Part model, mm, in its own coordinate system. A direction names the side the tool comes from. Give positions to 0.01 mm unless a question says otherwise; leave off trailing zeros. Write each loop counter-clockwise with the first axis right and the second up, starting at its lowest first coordinate (ties: lowest second). Pieces come first, ordered by that corner, then holes. Notation, with made-up numbers: (57, -34.5) - (74, -34.5) arc R16 cw to (74, -15.5) - close; hole circle Ø11 at (59.5, 86.5). An arc over 180 degrees is marked (long way). Answer in a Markdown table with one row per item. Add a question column.
1. Band-saw the part on D-D on z = 5. Write the cut outline in (x, y), plus the area to 3 significant figures.
2. Which spindle directions (+Z, -Z, +X, -X, +Y, -Y) get a long thin tool onto all of the face, cutting with end or side? Do faces 1 (the cylindrical face through (91.515, -6.601, 1.578)), 2 (the flat face through (83, -6, 5.8)). Say none if no direction does.
3. Drop flat-ended pins along their axis: pin 1 Ø1 at (x, y) = (89.5, -6.5) entering from -Z; pin 2 Ø3 at (y, z) = (-7.5, 3) entering from +X; pin 3 Ø3 at (y, z) = (-2.5, 2.5) entering from -X; pin 4 Ø6.5 at (x, y) = (85.21, -1.76) entering from +Z. Give the stop position or say it passes through.
4. Probe line 1 along X through (y, z) = (-1.75, 3.6); line 2 along Y through (x, z) = (84.25, 0.3); line 3 along X through (y, z) = (5.5, 1). List the from-to ranges inside material, lowest first.
5. Band-saw the part on C-C on z = 1.45. Write the cut outline in (x, y).
6. Pull direction Y, two halves, no side cores. Call faces 3 (the cylindrical face through (81.21, -1.59, 4.26)), 4 (the cylindrical face through (93.75, -5.31, 2.86)), 5 (the flat face through (88, 6, 0)): released by +Y, released by -Y, zero draft, split by the parting line, or undercut.
7. Band-saw the part on A-A on x = 79. Write the cut outline in (y, z).
8. Band-saw the part on B-B on y = 5.25. Write the cut outline in (x, z).
```python
from build123d import *

# Parameters (mm, degrees)
SKETCH1_R           = 9.25
BOSS_EXTRUDE1_DEPTH = 5.8
SKETCH2_R           = 4
CUT_EXTRUDE1_DEPTH  = 96.273205671
SKETCH3_R           = 7.95
CUT_EXTRUDE2_DEPTH  = 3.2
FILLET1_R           = 0.5


with BuildPart() as part:
    # Sketch1 → Boss-Extrude1 (new body)
    with BuildSketch(Plane.XY):
        with Locations((85.206527413, -1.763997815)):
            Circle(SKETCH1_R)
    extrude(amount=BOSS_EXTRUDE1_DEPTH)

    # Sketch2 → Cut-Extrude1 (cut, through all)
    with BuildSketch(Plane.XY.offset(5.8)):
        with Locations((85.206527413, -1.763997815)):
            Circle(SKETCH2_R)
    extrude(amount=-CUT_EXTRUDE1_DEPTH, mode=Mode.SUBTRACT)

    # Sketch3 → Cut-Extrude2 (cut)
    with BuildSketch(Plane(origin=(0, 0, 0), x_dir=(-1, 0, 0), z_dir=(0, 0, -1))):
        with Locations((-85.206527413, -1.763997815)):
            Circle(SKETCH3_R)
    extrude(amount=-CUT_EXTRUDE2_DEPTH, mode=Mode.SUBTRACT)

    # Fillet1
    fillet1_edges = [part.edges().sort_by_distance(p)[0] for p in [
        (81.206527413, -1.763997815, 5.8),
    ]]
    fillet(fillet1_edges, radius=FILLET1_R)


solid = part.part
```
Values:
| question | item | result |
|---|---|---|
| 1 | outline | circle Ø18.5 at (85.21, -1.76); hole circle Ø8 at (85.21, -1.76) |
| 1 | area | 219 mm² |
| 2 | face 1 | -Z |
| 2 | face 2 | +Z, +X, -X, +Y, -Y |
| 3 | pin 1 | stops at z = 3.2 |
| 3 | pin 2 | stops at x = 93.43 |
| 3 | pin 3 | stops at x = 75.96 |
| 3 | pin 4 | passes through |
| 4 | line 1 | x = 75.96 to 81.21, 89.21 to 94.46 |
| 4 | line 2 | y = -10.96 to -9.66, 6.13 to 7.44 |
| 4 | line 3 | x = 79.48 to 81.98, 88.44 to 90.93 |
| 5 | outline | circle Ø18.5 at (85.21, -1.76); hole circle Ø15.9 at (85.21, -1.76) |
| 6 | face 3 | undercut |
| 6 | face 4 | split by the parting line |
| 6 | face 5 | zero draft |
| 7 | outline | (-8.62, 0) - (-6.73, 0) - (-6.73, 3.2) - (3.2, 3.2) - (3.2, 0) - (5.09, 0) - (5.09, 5.8) - (-8.62, 5.8) - close |
| 8 | outline | (79.18, 0) - (81.46, 0) - (81.46, 3.2) - (88.95, 3.2) - (88.95, 0) - (91.24, 0) - (91.24, 5.8) - (79.18, 5.8) - close |
